Verification items for this drawing (mm, ordinates from the low corner). A direction names the side the tool comes from. Round coordinates to 2 decimals unless told otherwise and drop trailing zeros. Write each loop counter-clockwise with the first axis right and the second up, starting at its lowest first coordinate (ties: lowest second). Pieces come first, ordered by that corner, then holes. Notation, with made-up numbers: (74.25, 72.25) -> (120.25, 72.25) arc R25 cw to (120.25, 88.25) -> close; hole circle Ø6 at (75.5, -4). An arc over 180 degrees is marked (long way). One line per question, with ' | ' between items.
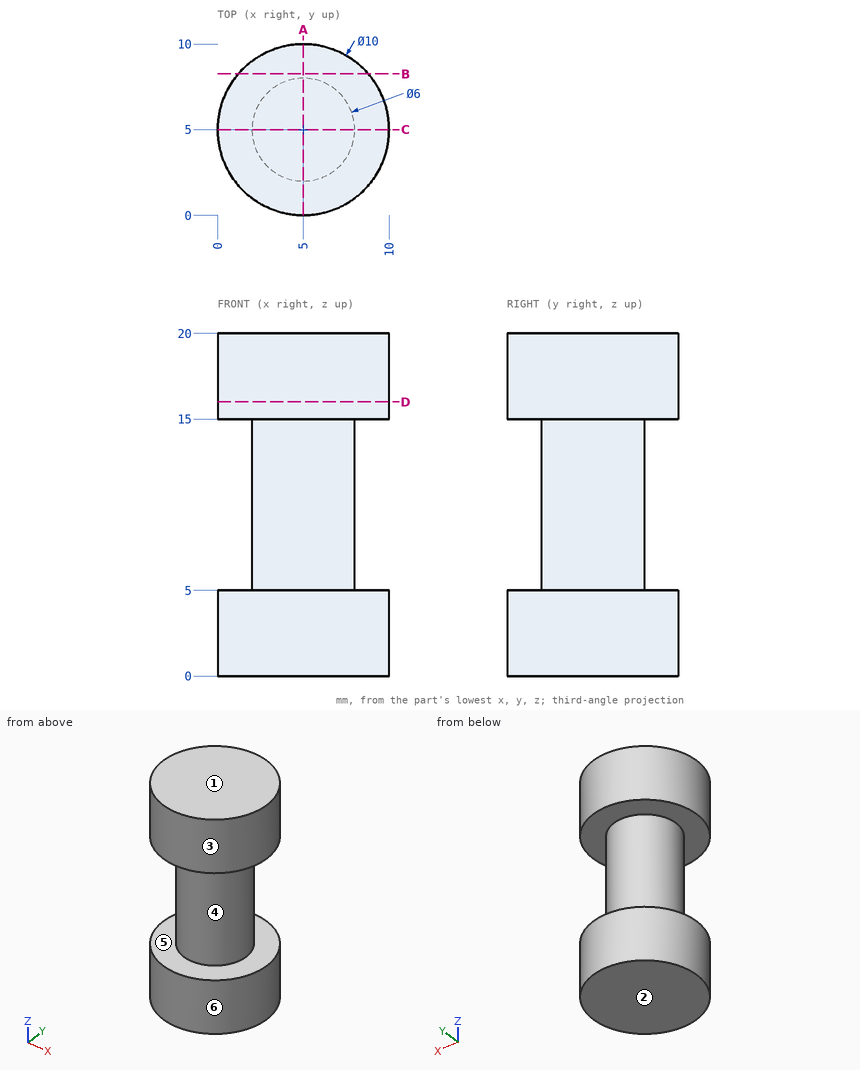
(1) Go/stop test with flat-tipped pins: pin 1 (5 mm diameter, centred on x = 2.5, z = 12, fed in from +Y); pin 2 (1.5 mm diameter, centred on x = 3.5, z = 5, fed in from +Y); pin 3 (2 mm diameter, centred on y = 8.5, z = 4.5, fed in from +X). Record where each tip stops, or that it passes through.
Resolved:
pin 1: stops at y = 8 | pin 2: stops at y = 9.94 | pin 3: stops at x = 9.33
(2) Draft check along Z on the marked faces 1, 2, 3 and 4. Enter one of: +Z half, -Z half, draft (parallel to the pull), parting line (faces both ways), or undercut.
Resolved:
face 1: +Z half | face 2: -Z half | face 3: draft | face 4: undercut
(3) Material ranges on line 1 (Z direction, x = 2, y = 6.75); line 2 (X direction, y = 6.5, z = 4); line 3 (Y direction, x = 9.5, z = 2.5), recorded low to high.
Resolved:
line 1: z = 0 to 5, 15 to 20 | line 2: x = 0.23 to 9.77 | line 3: y = 2.82 to 7.18
(4) Sectioned sample at A-A on x = 5. Record the cut outline in (y, z), then the cut area to 3 significant figures.
Resolved:
outline: (0, 0) -> (10, 0) -> (10, 5) -> (8, 5) -> (8, 15) -> (10, 15) -> (10, 20) -> (0, 20) -> (0, 15) -> (2, 15) -> (2, 5) -> (0, 5) -> close | area: 160 mm2
(5) Access from +Z, -Z, +X, -X, +Y, -Y to the whole of each face (thin tool, end or side, straight path). Record for the marked faces 5 and 6.
Resolved:
face 5: none | face 6: +Z, -Z
(6) Sectioned sample at B-B on y = 8.25. Record the cut outline in (x, z), then the cut area to 3 significant figures.
Resolved:
outline: (1.2, 0) -> (8.8, 0) -> (8.8, 5) -> (1.2, 5) -> close; (1.2, 15) -> (8.8, 15) -> (8.8, 20) -> (1.2, 20) -> close | area: 76.0 mm2
(7) Sectioned sample at D-D on z = 16. Record the cut outline in (x, y).
Resolved:
outline: circle Ø10 at (5, 5)
